Source: CAD feature listing. Evaluate the final solid. Frame: model axes, mm. A direction names the side the tool comes from. Give positions to 0.01 mm unless a question says otherwise; leave off trailing zeros. Order: outer loops, then holes, each group sorted by start corner. A loop starts at its lowest first (then second) coordinate and runs counter-clockwise, first axis right, second up. Notation, with made-up numbers: (60.25, -8) - (118.25, -8) arc R24 cw to (118.25, 24) - close; hole circle Ø4 at (-20.5, 5). An arc over 180 degrees is marked (long way). Write each question's results on one line, items separated by ' | '. Start each with the question number.
Item 1: Line query: line 1 along X through (y, z) = (40, -132); line 2 along Z through (x, y) = (7.5, 73); line 3 along Y through (x, z) = (-2, -133.25). Output: solid intervals per line, ascending.
Item 2: Set-up query: faces 1 (the conical face through (12.003, -1.973, -130.851)), 2 (the conical face through (35.351, 47.685, -132.837)), 3 (the flat face through (27, 6, -140.795)). Return all of +Z, -Z, +X, -X, +Y, -Y with unobstructed straight access to the full face (end or side cutting, diameter ignored); none if empty.
Item 3: Section A-A on z = -133. Output: boundary loops of the cut face in (x, y), and give its area (3 significant figures).
Item 4: Contact query for flat-ended pins moving along their axis: pin 1 Ø1 at (y, z) = (56, -135.5) entering from -X; pin 2 Ø5 at (y, z) = (38.5, -130) entering from -X; pin 3 Ø4 at (y, z) = (41, -138.5) entering from +X. Output: stop coordinate, or through.
```python
from build123d import *

# Parameters (mm, degrees)
SKETCH2_R                     = 49.197422353
BOSS_EXTRUDE1_DEPTH           = 9
BOSS_EXTRUDE1_TAPER           = 1.5
BOSS_EXTRUDE1_OTHER_WAY_DEPTH = 6
BOSS_EXTRUDE1_OTHER_WAY_TAPER = -1.5
SHELL1_T                      = -4
FILLET1_R                     = 5
SKETCH6_R                     = 13
WIREHOLES_DEPTH               = 10
WIREHOLES_DRAFT               = -1
SKETCH7_R                     = 48.404537882
INSIDELAYER_DEPTH             = 5
INSIDELAYER_DRAFT             = -1
SKETCH8_R                     = 1.500272091
NAIL_DEPTH                    = 10
NAIL_DRAFT                    = -1
SKETCH8_R_2                   = 1.501577836
NAIL_PROFILE_2_DEPTH          = 10
NAIL_PROFILE_2_DRAFT          = -1
SKETCH9_R                     = 3
NAILHEAD_DEPTH                = 2


with BuildPart() as part:
    # Sketch2 → Boss-Extrude1 (new body)
    with BuildSketch(Plane.XY.offset(-134.795498858)):
        with Locations((-8.948, 38.989)):
            Circle(SKETCH2_R)
    extrude(amount=BOSS_EXTRUDE1_DEPTH, taper=BOSS_EXTRUDE1_TAPER)

    # Sketch2 → Boss-Extrude1 other way (add)
    with BuildSketch(Plane.XY.offset(-134.795498858)):
        with Locations((-8.948, 38.989)):
            Circle(SKETCH2_R)
    extrude(amount=-BOSS_EXTRUDE1_OTHER_WAY_DEPTH, taper=BOSS_EXTRUDE1_OTHER_WAY_TAPER)

    # Shell1
    shell1_openings = [part.faces().sort_by_distance(p)[0] for p in [
        (-8.948, 38.989, -140.795498858),
    ]]
    offset(amount=SHELL1_T, openings=shell1_openings, kind=Kind.INTERSECTION)

    # Fillet1
    fillet1_edges = [part.edges().sort_by_distance(p)[0] for p in [
        (-57.909749059, 38.989, -125.795498858),
    ]]
    fillet(fillet1_edges, radius=FILLET1_R)


with BuildPart() as wireholes_tool:
    # Sketch6 → wireHoles (with draft: the straight prism first)
    with BuildSketch(Plane.XY.offset(-125.795498858)):
        with Locations((-37.201803, 40.335557149)):
            Circle(SKETCH6_R)
    extrude(amount=-WIREHOLES_DEPTH)
    # wireHoles: the draft: its side faces are tilted about the plane it starts from
    wireholes_sides = [wireholes_tool.faces().sort_by_distance(p)[0] for p in [
        (-50.201803, 40.335557149, -130.795498858),
    ]]
    draft(wireholes_sides, Plane.XY.offset(-125.795498858), WIREHOLES_DRAFT)


with BuildPart() as part_1:
    add(part.part)

    # wireHoles: cut by wireholes_tool
    add(wireholes_tool.part, mode=Mode.SUBTRACT)


with BuildPart() as insidelayer_tool:
    # Sketch7 → insideLayer (with draft: the straight prism first)
    with BuildSketch(Plane(origin=(0, 0, -140.795498858), x_dir=(-1, 0, 0), z_dir=(0, 0, -1))):
        with Locations((8.948, 38.989)):
            Circle(SKETCH7_R)
    extrude(amount=-INSIDELAYER_DEPTH)
    # insideLayer: the draft: its side faces are tilted about the plane it starts from
    insidelayer_sides = [insidelayer_tool.faces().sort_by_distance(p)[0] for p in [
        (39.456537882, 38.989, -138.295498858),
    ]]
    draft(insidelayer_sides, Plane(origin=(0, 0, -140.795498858), x_dir=(-1, 0, 0), z_dir=(0, 0, -1)), INSIDELAYER_DRAFT)


with BuildPart() as part_2:
    add(part_1.part)

    # insideLayer: cut by insidelayer_tool
    add(insidelayer_tool.part, mode=Mode.SUBTRACT)


with BuildPart() as nail_tool:
    # Sketch8 → nail (with draft: the straight prism first)
    with BuildSketch(Plane.XY.offset(-125.795498858)):
        with Locations((11.351812063, -0.720065293)):
            Circle(SKETCH8_R)
    extrude(amount=-NAIL_DEPTH)
    # nail: the draft: its side faces are tilted about the plane it starts from
    nail_sides = [nail_tool.faces().sort_by_distance(p)[0] for p in [
        (9.851539971, -0.720065293, -130.795498858),
    ]]
    draft(nail_sides, Plane.XY.offset(-125.795498858), NAIL_DRAFT)


with BuildPart() as part_3:
    add(part_2.part)

    # nail: cut by nail_tool
    add(nail_tool.part, mode=Mode.SUBTRACT)


with BuildPart() as nail_profile_2_tool:
    # Sketch8 → nail profile 2 (with draft: the straight prism first)
    with BuildSketch(Plane.XY.offset(-125.795498858)):
        with Locations((-6.787419008, 83.581267699)):
            Circle(SKETCH8_R_2)
    extrude(amount=-NAIL_PROFILE_2_DEPTH)
    # nail profile 2: the draft: its side faces are tilted about the plane it starts from
    nail_profile_2_sides = [nail_profile_2_tool.faces().sort_by_distance(p)[0] for p in [
        (-8.288996843, 83.581267699, -130.795498858),
    ]]
    draft(nail_profile_2_sides, Plane.XY.offset(-125.795498858), NAIL_PROFILE_2_DRAFT)


with BuildPart() as part_4:
    add(part_3.part)

    # nail profile 2: cut by nail_profile_2_tool
    add(nail_profile_2_tool.part, mode=Mode.SUBTRACT)

    # Sketch9 → nailHead (cut)
    with BuildSketch(Plane.XY.offset(-125.795498858)):
        with Locations((-6.787419008, 83.581267699)):
            Circle(SKETCH9_R)
        with Locations((11.351812063, -0.720065293)):
            Circle(SKETCH9_R)
    extrude(amount=-NAILHEAD_DEPTH, mode=Mode.SUBTRACT)


solid = part_4.part
```
Evaluation:
1) line 1: x = -58.06 to -54.06, 36.16 to 40.17 | line 2: z = -129.8 to -125.8 | line 3: y = -9.67 to -5.63, 83.61 to 87.65
2) face 1: +Z | face 2: -Z | face 3: -Z, +X, -X, +Y, -Y
3) outline: circle Ø98.3 at (-8.95, 38.99); hole (-8.05, 84.13) arc R45.15 ccw (long way) to (10.47, -1.77) arc R1.37 ccw to (12.72, -0.62) arc R45.15 ccw to (-5.48, 84) arc R1.38 ccw to start | area: 1,180 mm^2
4) pin 1: stops at x = -55.31 | pin 2: stops at x = -58.08 | pin 3: stops at x = 40.38
